Part model, mm, in its own coordinate system. A direction names the side the tool comes from. Round coordinates to 2 decimals unless told otherwise and drop trailing zeros. Order: outer loops, then holes, each group sorted by start corner. A loop starts at its lowest first (then second) coordinate and runs counter-clockwise, first axis right, second up. Notation, with made-up numbers: (87.5, 29) - (126.5, 29) arc R22 cw to (126.5, 48) - close; hole circle Ø11 at (32.25, -12.75). An arc over 180 degrees is marked (long way). Answer as a JSON object with one key per item and string values.
```python
from build123d import *

# Parameters (mm, degrees)
SKETCH1_R            = 8.492006583
SKETCH1_R_2          = 5.992006583
BOSS_EXTRUDE1_DEPTH  = 7.4
SKETCH2_R            = 8.492006583
BOSS_EXTRUDE2_DEPTH  = 1
CUT_EXTRUDE1_DEPTH   = 18.3
M3_CLEARANCE_HOLE1_D = 3.2


with BuildPart() as part:
    # Sketch1 → Boss-Extrude1 (new body)
    with BuildSketch(Plane.XY):
        with Locations((78.5761931, -343.7069923)):
            Circle(SKETCH1_R)
        with Locations((78.5761931, -343.7069923)):
            Circle(SKETCH1_R_2, mode=Mode.SUBTRACT)
    extrude(amount=BOSS_EXTRUDE1_DEPTH)

    # Sketch2 → Boss-Extrude2 (add)
    with BuildSketch(Plane.XY.offset(7.4)):
        with Locations((78.5761931, -343.7069923)):
            Circle(SKETCH2_R)
    extrude(amount=BOSS_EXTRUDE2_DEPTH)

    # Sketch3 → Cut-Extrude1 (cut)
    with BuildSketch(Plane(origin=(0, 0, 0), x_dir=(-1, 0, 0), z_dir=(0, 0, -1))):
        with BuildLine():
            Line((-84.785347699, -337.913843331), (-85.435569051, -348.713302055))
            ThreePointArc((-85.435569051, -348.713302055), (-87.052849272, -343.196623866), (-84.785347699, -337.913843331))
        make_face()
    extrude(amount=-CUT_EXTRUDE1_DEPTH, mode=Mode.SUBTRACT)

    # M3 Clearance Hole1 (through all)
    with Locations(Plane(origin=(0, 0, 7.4), x_dir=(-1, 0, 0), z_dir=(0, 0, -1))):
        with Locations((-78.5761931, -343.7069923)):
            Hole(M3_CLEARANCE_HOLE1_D / 2)


solid = part.part
```
Item 1: Tool access for faces 1 (the flat face through (80, -345, 7.4)), 2 (the flat face through (77.7, -345.5, 8.4)): list every direction of +Z, -Z, +X, -X, +Y, -Y with a clear straight run to the whole face (end or side of a thin tool).
Taken from the geometry:
{"face 1": "-Z", "face 2": "+Z, +X, -X, +Y, -Y"}
Item 2: Cut at D-D (y = -345.75). Write the cut outline in (x, z), plus the area to 3 significant figures.
Taken from the geometry:
{"outline": "(70.33, 0) - (72.94, 0) - (72.94, 7.4) - (84.21, 7.4) - (84.21, 0) - (85.26, 0) - (85.26, 8.4) - (70.33, 8.4) - close", "area": "42.0 mm2"}
Item 3: Probe L1, parallel to Z at x = 80.5, y = -346.5; L2, parallel to Y at x = 79, z = 1.25; L3, parallel to Y at x = 81.75, z = 7. List the from-to ranges inside material, lowest first. Write a range as from..to.
Taken from the geometry:
{"L1": "7.4..8.4", "L2": "-352.19..-349.68, -337.73..-335.23", "L3": "-351.58..-348.79, -338.62..-335.83"}
Item 4: Drop flat-ended pins along their axis: P1, Ø3, axis at x = 80.5, z = 1.5, coming from the +Y side; P2, Ø2.5, axis at x = 78.58, y = -343.71, coming from the +Z side; P3, Ø5, axis at y = -337, z = 1, coming from the -X side; P4, Ø4, axis at y = -347, z = 5.5, coming from the -X side. Give the stop position or say it passes through.
Taken from the geometry:
{"P1": "y = -335.23", "P2": "through", "P3": "x = 71.2", "P4": "x = 70.18"}
Item 5: Cut at B-B (x = 80.5). Write the cut outline in (y, z).
Taken from the geometry:
{"outline": "(-351.98, 0) - (-349.38, 0) - (-349.38, 7.4) - (-338.03, 7.4) - (-338.03, 0) - (-335.44, 0) - (-335.44, 8.4) - (-351.98, 8.4) - close"}
Item 6: Two-plate mould, pull along X, no slides. Class faces 3 (the flat face through (72.5, -345.5, 0)), 4 (the cylindrical face through (78.23, -345.27, 7.91)), 5 (the cylindrical face through (70.087, -343.926, 4.141)), 6 (the flat face through (85.106, -343.238, 4.141)): pulls with the +X half, pulls with the -X half, needs draft (parallel to the pull), parting line crosses it, or undercut.
Taken from the geometry:
{"face 3": "needs draft", "face 4": "undercut", "face 5": "parting line crosses it", "face 6": "pulls with the +X half"}
Item 7: Cut at C-C (x = 77.25). Write the cut outline in (y, z).
Taken from the geometry:
{"outline": "(-352.09, 0) - (-349.55, 0) - (-349.55, 7.4) - (-344.6, 7.4) - (-344.6, 8.4) - (-352.09, 8.4) - close; (-342.81, 7.4) - (-337.86, 7.4) - (-337.86, 0) - (-335.32, 0) - (-335.32, 8.4) - (-342.81, 8.4) - close"}
Item 8: Cut at A-A (y = -343). Write the cut outline in (x, z).
Taken from the geometry:
{"outline": "(70.11, 0) - (72.63, 0) - (72.63, 7.4) - (77.14, 7.4) - (77.14, 8.4) - (70.11, 8.4) - close; (80.01, 7.4) - (84.53, 7.4) - (84.53, 0) - (85.09, 0) - (85.09, 8.4) - (80.01, 8.4) - close"}
